The model under review builds one solid part; all positions refer to its coordinate system, in mm. A direction names the side the tool comes from. Give positions to 0.01 mm unless a question says otherwise; leave off trailing zeros. Loops run counter-clockwise (first coordinate to the right, second up) from the corner with the lowest first, then second, coordinate; pieces in that order, holes last. Notation, with made-up numbers: (9, -18) - (43, -18) arc R22 cw to (43, 4) - close; hole circle Ø11 at (-3.5, -23). An arc over 180 degrees is marked (long way). Answer as a JSON object with one key per item and string values.
from build123d import *

# Parameters (mm, degrees)
F0_R     = 2.157429
F0_R_2   = 5.60947
F1_DEPTH = 3.175
F0_R_3   = 2.141456
F2_DEPTH = 0.004921
F3_DEPTH = 3.175


with BuildPart() as f1:
    # F0 (on Front) → F1 (new body)
    with BuildSketch(Plane.XZ):
        with BuildLine():
            Line((19.481216, 38.301506), (-40.142396, 38.301506))
            ThreePointArc((-40.142396, 38.301506), (-42.607797, 37.803368), (-44.686392, 36.387111))
            ThreePointArc((-44.686392, 36.387111), (-46.052064, 34.274936), (-46.490546, 31.798229))
            Line((-46.490546, 31.798229), (-44.625234, 18.579618))
            ThreePointArc((-44.625234, 18.579618), (-43.776004, 17.017098), (-42.110151, 16.394528))
            Line((-42.110151, 16.394528), (21.620648, 16.394528))
            ThreePointArc((21.620648, 16.394528), (23.297675, 17.026865), (24.139706, 18.609033))
            Line((24.139706, 18.609033), (25.823629, 31.641185))
            ThreePointArc((25.823629, 31.641185), (24.07975, 36.330545), (19.481216, 38.301506))
        make_face()
        with Locations((-36.75957, 20.633117)):
            Circle(F0_R, mode=Mode.SUBTRACT)
        with BuildLine():
            Line((-29.799683, 20.633117), (-29.799683, 34.853889))
            ThreePointArc((-29.799683, 34.853889), (-27.878732, 36.660702), (-26.0331, 34.777018))
            Line((-26.0331, 34.777018), (-26.0331, 20.556246))
            ThreePointArc((-26.0331, 20.556246), (-27.954051, 18.749433), (-29.799683, 20.633117))
        make_face(mode=Mode.SUBTRACT)
        with BuildLine():
            Line((-24.176236, 20.709988), (-24.176236, 34.93076))
            ThreePointArc((-24.176236, 34.93076), (-22.255285, 36.737572), (-20.409653, 34.853889))
            Line((-20.409653, 34.853889), (-20.409653, 20.633116))
            ThreePointArc((-20.409653, 20.633116), (-22.330604, 18.826304), (-24.176236, 20.709988))
        make_face(mode=Mode.SUBTRACT)
        with BuildLine():
            Line((-18.419787, 20.786859), (-18.419787, 35.007631))
            ThreePointArc((-18.419787, 35.007631), (-16.498836, 36.814444), (-14.653204, 34.93076))
            Line((-14.653204, 34.93076), (-14.653204, 20.709988))
            ThreePointArc((-14.653204, 20.709988), (-16.574155, 18.903175), (-18.419787, 20.786859))
        make_face(mode=Mode.SUBTRACT)
        with Locations((17.996946, 20.940602)):
            Circle(F0_R, mode=Mode.SUBTRACT)
        with BuildLine():
            Line((-12.493486, 20.86373), (-12.493486, 35.084503))
            ThreePointArc((-12.493486, 35.084503), (-10.572535, 36.891315), (-8.726902, 35.007631))
            Line((-8.726902, 35.007631), (-8.726902, 20.786859))
            ThreePointArc((-8.726902, 20.786859), (-10.647853, 18.980047), (-12.493486, 20.86373))
        make_face(mode=Mode.SUBTRACT)
        with BuildLine():
            Line((-6.886294, 20.940602), (-6.886294, 35.161374))
            ThreePointArc((-6.886294, 35.161374), (-4.965343, 36.968187), (-3.11971, 35.084503))
            Line((-3.11971, 35.084503), (-3.11971, 20.86373))
            ThreePointArc((-3.11971, 20.86373), (-5.040661, 19.056918), (-6.886294, 20.940602))
        make_face(mode=Mode.SUBTRACT)
        with BuildLine():
            Line((-1.18931, 21.017473), (-1.18931, 35.238246))
            ThreePointArc((-1.18931, 35.238246), (0.73164, 37.045058), (2.577273, 35.161374))
            Line((2.577273, 35.161374), (2.577273, 20.940602))
            ThreePointArc((2.577273, 20.940602), (0.656322, 19.133789), (-1.18931, 21.017473))
        make_face(mode=Mode.SUBTRACT)
        with BuildLine():
            Line((4.431474, 21.017473), (4.431474, 35.238246))
            ThreePointArc((4.431474, 35.238246), (6.352424, 37.045058), (8.198057, 35.161374))
            Line((8.198057, 35.161374), (8.198057, 20.940602))
            ThreePointArc((8.198057, 20.940602), (6.277106, 19.133789), (4.431474, 21.017473))
        make_face(mode=Mode.SUBTRACT)
        with Locations((-38.274463, 31.951506)):
            Circle(F0_R_2, mode=Mode.SUBTRACT)
        with Locations((17.949626, 31.951506)):
            Circle(F0_R_2, mode=Mode.SUBTRACT)
    extrude(amount=F1_DEPTH)

    # F0 (on Front) → F2 (join)
    with BuildSketch(Plane.XZ):
        with BuildLine():
            Line((19.481216, 38.301506), (-40.142396, 38.301506))
            ThreePointArc((-40.142396, 38.301506), (-42.607797, 37.803368), (-44.686392, 36.387111))
            ThreePointArc((-44.686392, 36.387111), (-46.052064, 34.274936), (-46.490546, 31.798229))
            Line((-46.490546, 31.798229), (-44.625234, 18.579618))
            ThreePointArc((-44.625234, 18.579618), (-43.776004, 17.017098), (-42.110151, 16.394528))
            Line((-42.110151, 16.394528), (21.620648, 16.394528))
            ThreePointArc((21.620648, 16.394528), (23.297675, 17.026865), (24.139706, 18.609033))
            Line((24.139706, 18.609033), (25.823629, 31.641185))
            ThreePointArc((25.823629, 31.641185), (24.07975, 36.330545), (19.481216, 38.301506))
        make_face()
        with Locations((-36.75957, 20.633117)):
            Circle(F0_R, mode=Mode.SUBTRACT)
        with BuildLine():
            Line((-29.799683, 20.633117), (-29.799683, 34.853889))
            ThreePointArc((-29.799683, 34.853889), (-27.878732, 36.660702), (-26.0331, 34.777018))
            Line((-26.0331, 34.777018), (-26.0331, 20.556246))
            ThreePointArc((-26.0331, 20.556246), (-27.954051, 18.749433), (-29.799683, 20.633117))
        make_face(mode=Mode.SUBTRACT)
        with BuildLine():
            Line((-24.176236, 20.709988), (-24.176236, 34.93076))
            ThreePointArc((-24.176236, 34.93076), (-22.255285, 36.737572), (-20.409653, 34.853889))
            Line((-20.409653, 34.853889), (-20.409653, 20.633116))
            ThreePointArc((-20.409653, 20.633116), (-22.330604, 18.826304), (-24.176236, 20.709988))
        make_face(mode=Mode.SUBTRACT)
        with BuildLine():
            Line((-18.419787, 20.786859), (-18.419787, 35.007631))
            ThreePointArc((-18.419787, 35.007631), (-16.498836, 36.814444), (-14.653204, 34.93076))
            Line((-14.653204, 34.93076), (-14.653204, 20.709988))
            ThreePointArc((-14.653204, 20.709988), (-16.574155, 18.903175), (-18.419787, 20.786859))
        make_face(mode=Mode.SUBTRACT)
        with Locations((17.996946, 20.940602)):
            Circle(F0_R, mode=Mode.SUBTRACT)
        with BuildLine():
            Line((-12.493486, 20.86373), (-12.493486, 35.084503))
            ThreePointArc((-12.493486, 35.084503), (-10.572535, 36.891315), (-8.726902, 35.007631))
            Line((-8.726902, 35.007631), (-8.726902, 20.786859))
            ThreePointArc((-8.726902, 20.786859), (-10.647853, 18.980047), (-12.493486, 20.86373))
        make_face(mode=Mode.SUBTRACT)
        with BuildLine():
            Line((-6.886294, 20.940602), (-6.886294, 35.161374))
            ThreePointArc((-6.886294, 35.161374), (-4.965343, 36.968187), (-3.11971, 35.084503))
            Line((-3.11971, 35.084503), (-3.11971, 20.86373))
            ThreePointArc((-3.11971, 20.86373), (-5.040661, 19.056918), (-6.886294, 20.940602))
        make_face(mode=Mode.SUBTRACT)
        with BuildLine():
            Line((-1.18931, 21.017473), (-1.18931, 35.238246))
            ThreePointArc((-1.18931, 35.238246), (0.73164, 37.045058), (2.577273, 35.161374))
            Line((2.577273, 35.161374), (2.577273, 20.940602))
            ThreePointArc((2.577273, 20.940602), (0.656322, 19.133789), (-1.18931, 21.017473))
        make_face(mode=Mode.SUBTRACT)
        with BuildLine():
            Line((4.431474, 21.017473), (4.431474, 35.238246))
            ThreePointArc((4.431474, 35.238246), (6.352424, 37.045058), (8.198057, 35.161374))
            Line((8.198057, 35.161374), (8.198057, 20.940602))
            ThreePointArc((8.198057, 20.940602), (6.277106, 19.133789), (4.431474, 21.017473))
        make_face(mode=Mode.SUBTRACT)
        with Locations((-38.274463, 31.951506)):
            Circle(F0_R_2, mode=Mode.SUBTRACT)
        with Locations((17.949626, 31.951506)):
            Circle(F0_R_2, mode=Mode.SUBTRACT)
        with BuildLine():
            ThreePointArc((-46.490546, 31.798229), (-46.052064, 34.274936), (-44.686392, 36.387111))
            ThreePointArc((-44.686392, 36.387111), (-50.775954, 38.77664), (-48.483074, 32.650033))
            ThreePointArc((-48.483074, 32.650033), (-47.542505, 32.09385), (-46.490546, 31.798229))
        make_face()
        with Locations((-48.263825, 36.469538)):
            Circle(F0_R_3, mode=Mode.SUBTRACT)
    extrude(amount=F2_DEPTH)

    # F0 (on Front) → F3 (join)
    with BuildSketch(Plane.XZ):
        with BuildLine():
            Line((19.481216, 38.301506), (-40.142396, 38.301506))
            ThreePointArc((-40.142396, 38.301506), (-42.607797, 37.803368), (-44.686392, 36.387111))
            ThreePointArc((-44.686392, 36.387111), (-46.052064, 34.274936), (-46.490546, 31.798229))
            Line((-46.490546, 31.798229), (-44.625234, 18.579618))
            ThreePointArc((-44.625234, 18.579618), (-43.776004, 17.017098), (-42.110151, 16.394528))
            Line((-42.110151, 16.394528), (21.620648, 16.394528))
            ThreePointArc((21.620648, 16.394528), (23.297675, 17.026865), (24.139706, 18.609033))
            Line((24.139706, 18.609033), (25.823629, 31.641185))
            ThreePointArc((25.823629, 31.641185), (24.07975, 36.330545), (19.481216, 38.301506))
        make_face()
        with Locations((-36.75957, 20.633117)):
            Circle(F0_R, mode=Mode.SUBTRACT)
        with BuildLine():
            Line((-29.799683, 20.633117), (-29.799683, 34.853889))
            ThreePointArc((-29.799683, 34.853889), (-27.878732, 36.660702), (-26.0331, 34.777018))
            Line((-26.0331, 34.777018), (-26.0331, 20.556246))
            ThreePointArc((-26.0331, 20.556246), (-27.954051, 18.749433), (-29.799683, 20.633117))
        make_face(mode=Mode.SUBTRACT)
        with BuildLine():
            Line((-24.176236, 20.709988), (-24.176236, 34.93076))
            ThreePointArc((-24.176236, 34.93076), (-22.255285, 36.737572), (-20.409653, 34.853889))
            Line((-20.409653, 34.853889), (-20.409653, 20.633116))
            ThreePointArc((-20.409653, 20.633116), (-22.330604, 18.826304), (-24.176236, 20.709988))
        make_face(mode=Mode.SUBTRACT)
        with BuildLine():
            Line((-18.419787, 20.786859), (-18.419787, 35.007631))
            ThreePointArc((-18.419787, 35.007631), (-16.498836, 36.814444), (-14.653204, 34.93076))
            Line((-14.653204, 34.93076), (-14.653204, 20.709988))
            ThreePointArc((-14.653204, 20.709988), (-16.574155, 18.903175), (-18.419787, 20.786859))
        make_face(mode=Mode.SUBTRACT)
        with Locations((17.996946, 20.940602)):
            Circle(F0_R, mode=Mode.SUBTRACT)
        with BuildLine():
            Line((-12.493486, 20.86373), (-12.493486, 35.084503))
            ThreePointArc((-12.493486, 35.084503), (-10.572535, 36.891315), (-8.726902, 35.007631))
            Line((-8.726902, 35.007631), (-8.726902, 20.786859))
            ThreePointArc((-8.726902, 20.786859), (-10.647853, 18.980047), (-12.493486, 20.86373))
        make_face(mode=Mode.SUBTRACT)
        with BuildLine():
            Line((-6.886294, 20.940602), (-6.886294, 35.161374))
            ThreePointArc((-6.886294, 35.161374), (-4.965343, 36.968187), (-3.11971, 35.084503))
            Line((-3.11971, 35.084503), (-3.11971, 20.86373))
            ThreePointArc((-3.11971, 20.86373), (-5.040661, 19.056918), (-6.886294, 20.940602))
        make_face(mode=Mode.SUBTRACT)
        with BuildLine():
            Line((-1.18931, 21.017473), (-1.18931, 35.238246))
            ThreePointArc((-1.18931, 35.238246), (0.73164, 37.045058), (2.577273, 35.161374))
            Line((2.577273, 35.161374), (2.577273, 20.940602))
            ThreePointArc((2.577273, 20.940602), (0.656322, 19.133789), (-1.18931, 21.017473))
        make_face(mode=Mode.SUBTRACT)
        with BuildLine():
            Line((4.431474, 21.017473), (4.431474, 35.238246))
            ThreePointArc((4.431474, 35.238246), (6.352424, 37.045058), (8.198057, 35.161374))
            Line((8.198057, 35.161374), (8.198057, 20.940602))
            ThreePointArc((8.198057, 20.940602), (6.277106, 19.133789), (4.431474, 21.017473))
        make_face(mode=Mode.SUBTRACT)
        with Locations((-38.274463, 31.951506)):
            Circle(F0_R_2, mode=Mode.SUBTRACT)
        with Locations((17.949626, 31.951506)):
            Circle(F0_R_2, mode=Mode.SUBTRACT)
        with BuildLine():
            ThreePointArc((-46.490546, 31.798229), (-46.052064, 34.274936), (-44.686392, 36.387111))
            ThreePointArc((-44.686392, 36.387111), (-50.775954, 38.77664), (-48.483074, 32.650033))
            ThreePointArc((-48.483074, 32.650033), (-47.542505, 32.09385), (-46.490546, 31.798229))
        make_face()
        with Locations((-48.263825, 36.469538)):
            Circle(F0_R_3, mode=Mode.SUBTRACT)
    extrude(amount=F3_DEPTH)


solid = f1.part
Q1. Clearance check with flat-ended pins moving along their axes: pin 1 Ø1 at (y, z) = (-1, 26.5) entering from -X; pin 2 Ø9 at (x, z) = (-38.27, 31.95) entering from +Y; pin 3 Ø1.6 at (y, z) = (-1.5, 25) entering from -X; pin 4 Ø1.6 at (y, z) = (-1, 30.5) entering from -X. State where each tip first meets the part, or that it passes through.
Results:
{"pin 1": "stops at x = -45.81", "pin 2": "passes through", "pin 3": "stops at x = -45.64", "pin 4": "stops at x = -46.42"}
Q2. To check wall thickness, follow probe 1 along Z at (x, y) = (-35, -1.85); probe 2 along Z at (x, y) = (-18, -2); probe 3 along Z at (x, y) = (-15, -2.9). State the ranges of each line that lie inside material, in increasing order. Write a range as [from, to].
Results:
{"probe 1": "z = [16.39, 19.38], [21.88, 27.4], [36.51, 38.3]", "probe 2": "z = [16.39, 19.6], [36.12, 38.3]", "probe 3": "z = [16.39, 19.7], [36.02, 38.3]"}
Q3. Consider section C-C, the plane y = -1.75. State how many separate pieces and enclosed holes the cut face has, plus the area to 3 significant figures.
Results:
{"separate pieces": "1", "enclosed holes": "12", "area": "881 mm^2"}
Q4. The part is to be moulded in two halves that separate along X. For faces 1 (the face through (-14, 0, 26)), 2 (the face through (2.577, -2, 28)), 3 (the face through (6.318, -1.565, 19.133)), 4 (the face through (23.28, -1.57, 17.01)), say which applies: +X half, -X half, draft (parallel to the pull), parting line (faces both ways), or undercut.
Results:
{"face 1": "draft", "face 2": "undercut", "face 3": "undercut", "face 4": "+X half"}
Q5. Consider section D-D, the plane x = -4.5. State the section outline as (y, z) points (1 decimal), plus the area to 3 significant figures.
Results:
{"outline": "(-3.2, 16.4) - (0, 16.4) - (0, 19.1) - (-3.2, 19.1) - close; (-3.2, 36.9) - (0, 36.9) - (0, 38.3) - (-3.2, 38.3) - close", "area": "13.1 mm^2"}
Q6. Consider section B-B, the plane x = -36. State the section outline as (y, z) points (1 decimal), plus the area to 3 significant figures.
Results:
{"outline": "(-3.2, 16.4) - (0, 16.4) - (0, 18.6) - (-3.2, 18.6) - close; (-3.2, 22.7) - (0, 22.7) - (0, 26.8) - (-3.2, 26.8) - close; (-3.2, 37.1) - (0, 37.1) - (0, 38.3) - (-3.2, 38.3) - close", "area": "24.2 mm^2"}
Q7. For faces 5 (the face through (-18.42, -2, 28)), 6 (the face through (-47.56, -1.57, 32.1)), list the 3-axis set-ups (+Z, -Z, +X, -X, +Y, -Y) from which the entire face can be reached by the end or side of a thin tool; tool diameter is ignored.
Results:
{"face 5": "+Y, -Y", "face 6": "-Z, -X, +Y, -Y"}
Q8. Consider section A-A, the plane x = -23. State the section outline as (y, z) points (1 decimal), plus the area to 3 significant figures.
Results:
{"outline": "(-3.2, 16.4) - (0, 16.4) - (0, 19) - (-3.2, 19) - close; (-3.2, 36.6) - (0, 36.6) - (0, 38.3) - (-3.2, 38.3) - close", "area": "13.6 mm^2"}
